Could you check a few things on this model? Use its own coordinates, in mm. Give positions to 0.01 mm unless a question says otherwise; leave off trailing zeros. Loops run counter-clockwise (first coordinate to the right, second up) from the corner with the lowest first, then second, coordinate; pieces in that order, holes last.
1. I need wall thicknesses on line 1 along X through (y, z) = (-64.5, -5); line 2 along X through (y, z) = (-94, -3.25); line 3 along Y through (x, z) = (1623, 2). Which ranges of each line are inside material? Lowest first, please.
2. Imagine slicing it at C-C (x = 1655.5). List the corners of the cut face in (y, z) for me.
3. Imagine slicing it at B-B (y = -217). List the corners of the cut face in (x, z) for me.
4. Imagine slicing it at D-D (y = -79.5). List the corners of the cut face in (x, z) for me.
5. Imagine slicing it at A-A (x = 1628). List the corners of the cut face in (y, z) for me.
6. For P1, Ø5, axis at x = 1689, z = 2.5, coming from the +Y side; P2, Ø1, axis at x = 1573, z = -1, coming from the +Y side; P3, Ø4, axis at y = -209, z = 3, coming from the -X side; P4, Ø7.5, axis at x = 1568.11, y = -30.78, coming from the -Z side, each with a flat end and sliding along its axis, tell me the tip position at first contact or that it passes through.
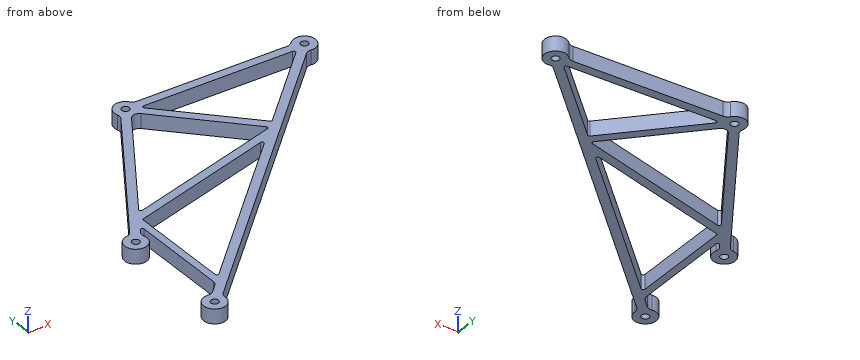
```python
from build123d import *

# Parameters (mm, degrees)
SKETCH1_R           = 3.2639
BOSS_EXTRUDE1_DEPTH = 6.35
FILLET1_R           = 6.35
FILLET2_R           = 1.524
FILLET3_R           = 5.715


with BuildPart() as part:
    # Sketch1 → Boss-Extrude1 (new, symmetric)
    with BuildSketch(Plane.XY):
        with BuildLine():
            Line((1487.79576568, -158.784269308), (1487.79576568, -250.194499736))
            Line((1487.79576568, -250.194499736), (1477.101010284, -260.227049093))
            ThreePointArc((1477.101010284, -260.227049093), (1466.258468724, -275.622237688), (1482.314360626, -265.784510583))
            Line((1482.314360626, -265.784510583), (1716.673663322, -45.936446331))
            ThreePointArc((1716.673663322, -45.936446331), (1729.515779421, -33.768446492), (1711.843687849, -32.945436509))
            Line((1711.843687849, -32.945436509), (1577.08389596, -27.343328807))
            ThreePointArc((1577.08389596, -27.343328807), (1563.736723174, -22.220026544), (1560.05306912, -36.03400281))
            Line((1560.05306912, -36.03400281), (1474.973065059, -164.332851502))
            ThreePointArc((1474.973065059, -164.332851502), (1467.95688272, -181.806995965), (1481.323608223, -168.54414602))
            Line((1481.323608223, -168.54414602), (1487.79576568, -158.784269308))
        make_face()
        with Locations((1473.270132637, -269.04472734)):
            Circle(SKETCH1_R, mode=Mode.SUBTRACT)
        with Locations((1473.270132637, -173.79472734)):
            Circle(SKETCH1_R, mode=Mode.SUBTRACT)
        Polygon((1494.14576568, -153.132601519), (1625.870376064, -120.66929862), (1494.14576568, -244.23768389), align=None, mode=Mode.SUBTRACT)
        with BuildLine():
            Line((1571.366761462, -39.827649479), (1637.217429421, -110.024840786))
            Line((1637.217429421, -110.024840786), (1497.256271331, -144.518026652))
            Line((1497.256271331, -144.518026652), (1566.403612284, -40.245297328))
            ThreePointArc((1566.403612284, -40.245297328), (1568.912702914, -40.363462312), (1571.366761462, -39.827649479))
        make_face(mode=Mode.SUBTRACT)
        with Locations((1568.106544706, -30.78342149)):
            Circle(SKETCH1_R, mode=Mode.SUBTRACT)
        Polygon((1642.774890911, -104.811490444), (1577.264872597, -34.97743362), (1711.279538853, -40.548565657), align=None, mode=Mode.SUBTRACT)
        with Locations((1720.504540969, -37.118768084)):
            Circle(SKETCH1_R, mode=Mode.SUBTRACT)
    extrude(amount=BOSS_EXTRUDE1_DEPTH, both=True)

    # Fillet1
    fillet1_edges = [part.edges().sort_by_distance(p)[0] for p in [
        (1577.08389596, -27.343328807, 0),
        (1711.843687849, -32.945436509, 0),
        (1716.673663322, -45.936446331, 0),
        (1482.314360626, -265.784510583, 0),
        (1477.101010284, -260.227049093, 0),
        (1487.79576568, -250.194499736, 0),
        (1481.323608223, -168.54414602, 0),
        (1474.973065059, -164.332851502, 0),
        (1560.05306912, -36.03400281, 0),
    ]]
    fillet(fillet1_edges, radius=FILLET1_R)

    # Fillet2
    fillet2_edges = [part.edges().sort_by_distance(p)[0] for p in [
        (1494.14576568, -244.23768389, 0),
        (1625.870376064, -120.66929862, 0),
        (1494.14576568, -153.132601519, 0),
        (1642.774890911, -104.811490444, 0),
        (1711.279538853, -40.548565657, 0),
        (1577.264872597, -34.97743362, 0),
        (1497.256271331, -144.518026652, 0),
        (1637.217429421, -110.024840786, 0),
        (1487.79576568, -158.784269308, 0),
    ]]
    fillet(fillet2_edges, radius=FILLET2_R)

    # Fillet3
    fillet3_edges = [part.edges().sort_by_distance(p)[0] for p in [
        (1571.366761462, -39.827649479, 0),
    ]]
    fillet(fillet3_edges, radius=FILLET3_R)
    fillet3_2_edges = [part.edges().sort_by_distance(p)[0] for p in [
        (1566.403612284, -40.245297328, 0),
    ]]
    fillet(fillet3_2_edges, radius=FILLET3_R - 0.0001)  # a hair under: the kernel refuses the full size


solid = part.part
```
Derived:
1. line 1: x = 1541.18 to 1550.32, 1594.51 to 1604.96, 1685.75 to 1696.88
1. line 2: x = 1521.61 to 1530.76, 1622.18 to 1632.63, 1654.3 to 1665.44
1. line 3: y = -133.81 to -113.53, -94.87 to -83.73, -36.88 to -29.25
2. outline: (-103.32, -6.35) - (-92.87, -6.35) - (-92.87, 6.35) - (-103.32, 6.35) - close; (-38.23, -6.35) - (-30.6, -6.35) - (-30.6, 6.35) - (-38.23, 6.35) - close
3. outline: (1487.8, -6.35) - (1494.15, -6.35) - (1494.15, 6.35) - (1487.8, 6.35) - close; (1523.18, -6.35) - (1534.32, -6.35) - (1534.32, 6.35) - (1523.18, 6.35) - close
4. outline: (1531.23, -6.35) - (1540.37, -6.35) - (1540.37, 6.35) - (1531.23, 6.35) - close; (1608.58, -6.35) - (1619.03, -6.35) - (1619.03, 6.35) - (1608.58, 6.35) - close; (1669.76, -6.35) - (1680.89, -6.35) - (1680.89, 6.35) - (1669.76, 6.35) - close
5. outline: (-129.12, -6.35) - (-112.3, -6.35) - (-112.3, 6.35) - (-129.12, 6.35) - close; (-100.2, -6.35) - (-89.06, -6.35) - (-89.06, 6.35) - (-100.2, 6.35) - close; (-37.09, -6.35) - (-29.46, -6.35) - (-29.46, 6.35) - (-37.09, 6.35) - close
6. P1: stops at y = -31.89
6. P2: stops at y = -22.23
6. P3: stops at x = 1487.8
6. P4: stops at z = -6.35
